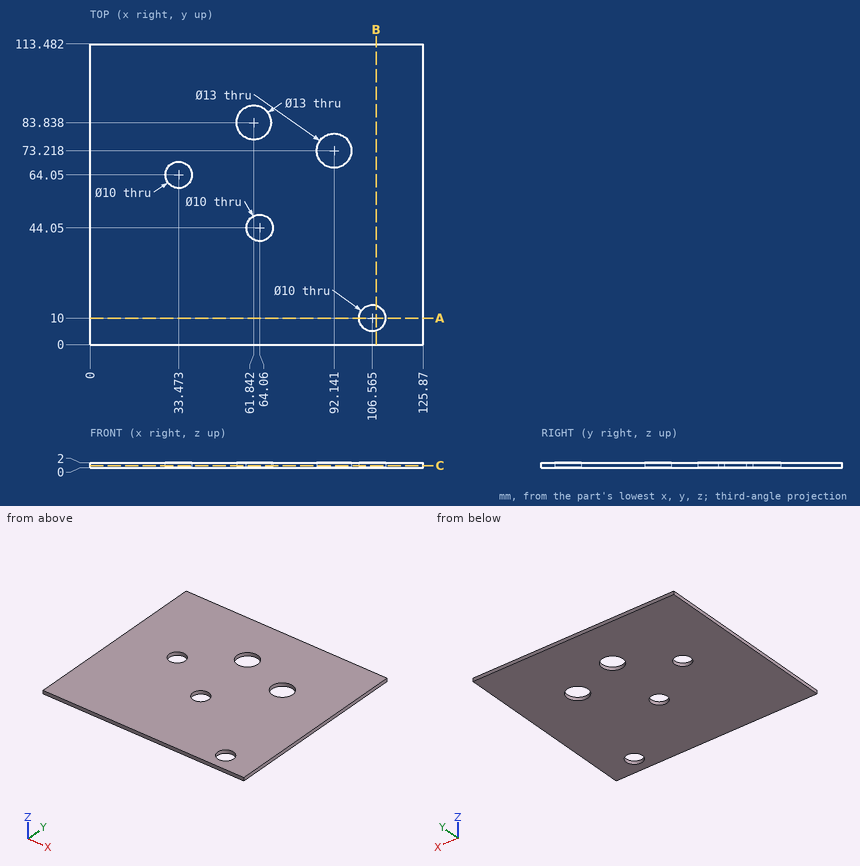
Here's the drawing with two shaded views (mm, measured from the low corner). I have some questions. Round coordinates to 2 decimals unless told otherwise and drop trailing zeros. Write each loop counter-clockwise with the first axis right and the second up, starting at its lowest first coordinate (ties: lowest second). Pieces come first, ordered by that corner, then holes. Notation, with made-up numbers: M -22.75,6 L 9.25,6 A19 ccw 9.25,24 Z; hole C -37,55.5 d1. An arc over 180 degrees is marked long. Answer in a Markdown table with one row per item. Add a question column.
Q1. If I drill on line 1 (X direction, y = 62, z = 1.3) (1 decimal); line 2 (X direction, y = 62.5, z = 0.45); line 3 (Y direction, x = 35.5, z = 1.75), over which ranges is the centre line in solid material (lowest first)? Write a range as from..to.
Q2. Will this pin go through, and if not, where does the flat tip stop? pin 1 Ø6 at (x, y) = (106.57, 10) entering from +Z.
Q3. Imagine slicing it at B-B (x = 108). Please give me the cut outline in (y, z), then the cut area to 3 significant figures.
Q4. Imagine slicing it at C-C (z = 0.9). Give the number of separate pieces and of enclosed holes in the cut face, then the cut area to 3 significant figures.
Q5. Imagine slicing it at A-A (y = 10). Please give me the cut outline in (x, z) (1 decimal), then the cut area to 3 significant figures.
Values:
| question | item | result |
|---|---|---|
| 1 | line 1 | 0..28.9, 38..125.9 |
| 1 | line 2 | 0..28.72, 38.23..125.87 |
| 1 | line 3 | 0..59.48, 68.62..113.48 |
| 2 | pin 1 | through |
| 3 | outline | M 0,0 L 5.21,0 L 5.21,2 L 0,2 Z; M 14.79,0 L 113.48,0 L 113.48,2 L 14.79,2 Z |
| 3 | area | 208 mm^2 |
| 4 | separate pieces | 1 |
| 4 | enclosed holes | 5 |
| 4 | area | 13,800 mm^2 |
| 5 | outline | M 0,0 L 101.6,0 L 101.6,2 L 0,2 Z; M 111.6,0 L 125.9,0 L 125.9,2 L 111.6,2 Z |
| 5 | area | 232 mm^2 |
